Drawing for the job (mm, zero at the part's lowest x, y, z). A direction names the side the tool comes from. Give positions to 0.01 mm unless a question says otherwise; leave off trailing zeros. Loops run counter-clockwise (first coordinate to the right, second up) from the corner with the lowest first, then second, coordinate; pieces in that order, holes last.
1) Flat gauge pins, fed straight in: P1, Ø5, axis at x = 42.5, z = 6.5, coming from the +Y side; P2, Ø6.5, axis at y = 14.25, z = 25, coming from the +X side; P3, Ø2.5, axis at x = 45, z = 25, coming from the -Y side; P4, Ø6, axis at y = 5.5, z = 16.5, coming from the -X side (1 decimal). Where does each tip first touch, or does it go through?
2) Band-saw the part on B-B on z = 5. List the corners of the cut face in (x, y).
3) Band-saw the part on D-D on y = 20.25. List the corners of the cut face in (x, z).
4) 3-axis set-ups, long thin cutter, end or side, ignore diameter. For the marked faces 1 and 2: which of +Z, -Z, +X, -X, +Y, -Y reach the whole face in a straight line?
5) Wall check: line 1 (Y direction, x = 36, z = 25) (1 decimal); line 2 (Z direction, x = 25.5, y = 10.75); line 3 (X direction, y = 10.25, z = 25). Give the ranges that are in metal, low to high.
6) Band-saw the part on A-A on x = 45. List the corners of the cut face in (y, z).
7) Band-saw the part on C-C on z = 25. List the corners of the cut face in (x, y) (1 decimal), then the cut area to 3 significant figures.
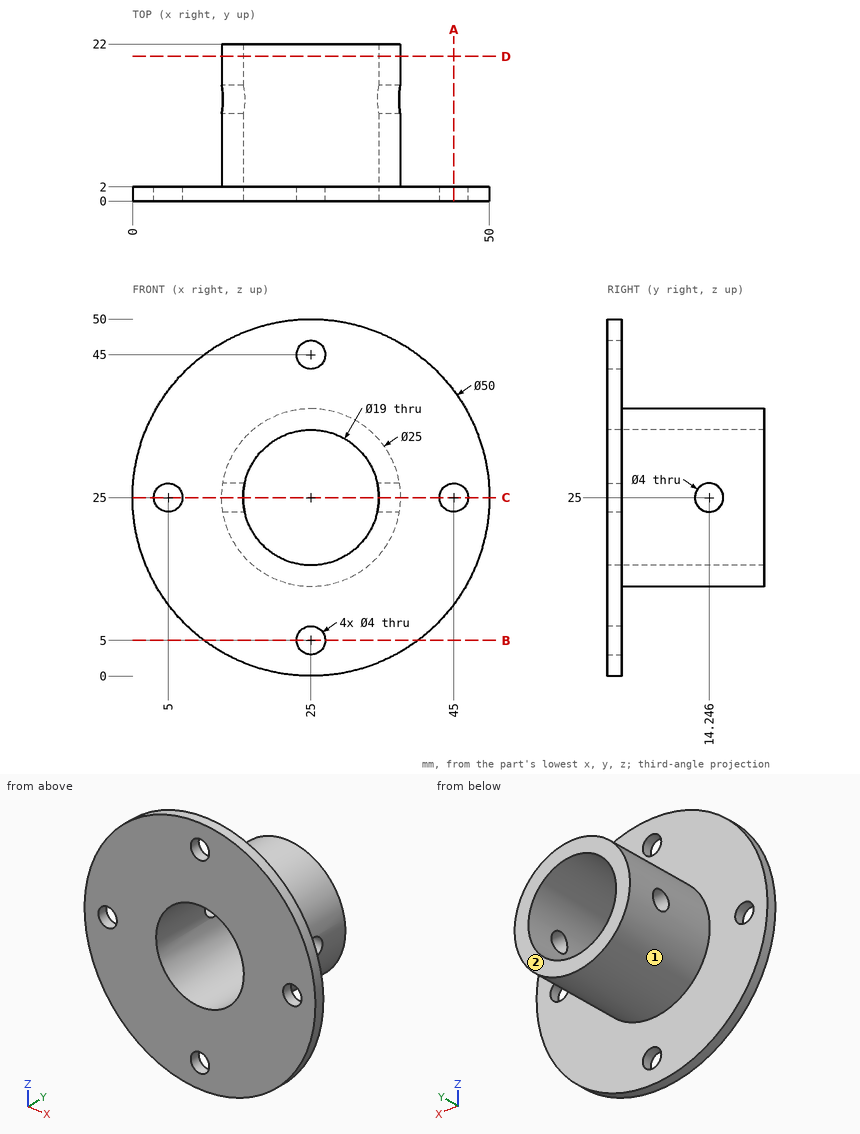
Findings below:
1. P1: stops at y = 2
1. P2: stops at x = 37.5
1. P3: passes through
1. P4: stops at x = 13.8
2. outline: (10, 0) - (23, 0) - (23, 2) - (10, 2) - close; (27, 0) - (40, 0) - (40, 2) - (27, 2) - close
3. outline: circle Ø25 at (25, 25); hole circle Ø19 at (25, 25)
4. face 1: +Y
4. face 2: +Z, -Z, +X, -X, +Y
5. line 1: y = 0 to 12.2, 16.2 to 22
5. line 2: z = 12.51 to 15.51, 34.49 to 37.49
5. line 3: x = 12.5 to 15.5, 34.5 to 37.5
6. outline: (0, 10) - (2, 10) - (2, 23) - (0, 23) - close; (0, 27) - (2, 27) - (2, 40) - (0, 40) - close
7. outline: (0, 0) - (3, 0) - (3, 2) - (0, 2) - close; (7, 0) - (15.5, 0) - (15.5, 12.2) - (12.5, 12.2) - (12.5, 2) - (7, 2) - close; (12.5, 16.2) - (15.5, 16.2) - (15.5, 22) - (12.5, 22) - close; (34.5, 0) - (43, 0) - (43, 2) - (37.5, 2) - (37.5, 12.2) - (34.5, 12.2) - close; (34.5, 16.2) - (37.5, 16.2) - (37.5, 22) - (34.5, 22) - close; (47, 0) - (50, 0) - (50, 2) - (47, 2) - close
7. area: 142 mm2
